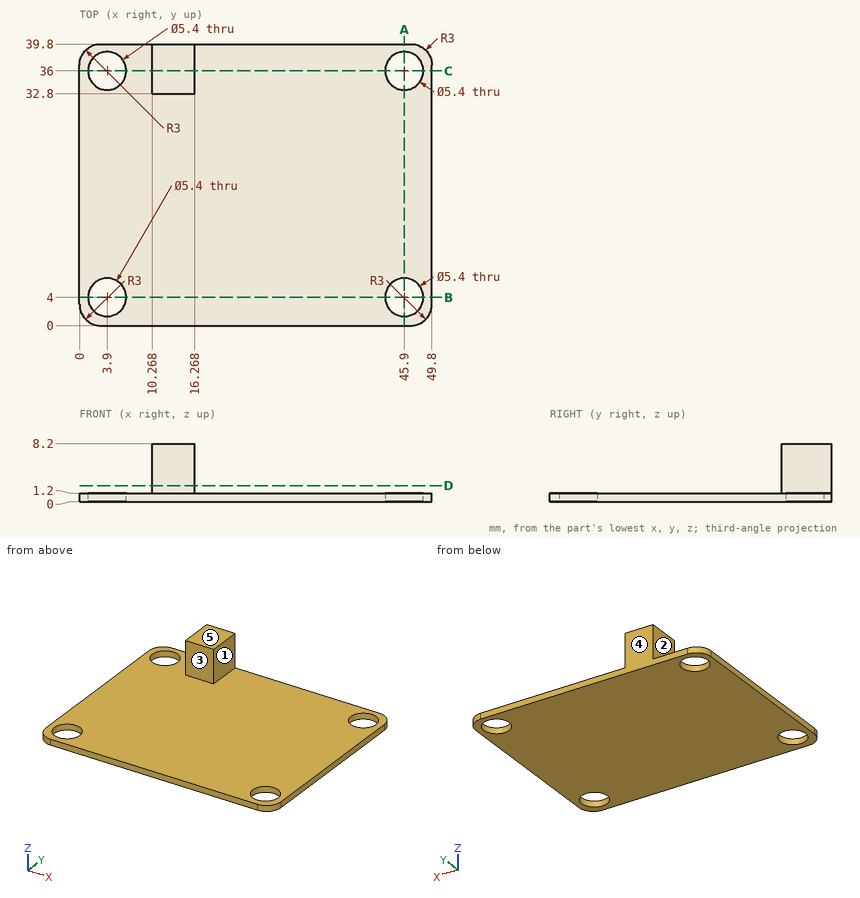
Source: three-view drawing plus pictorial views. Frame: mm from the lowest corner of the part. A direction names the side the tool comes from. Give positions to 0.01 mm unless a question says otherwise; leave off trailing zeros. Order: outer loops, then holes, each group sorted by start corner. A loop starts at its lowest first (then second) coordinate and runs counter-clockwise, first axis right, second up. Notation, with made-up numbers: (31, 89) -> (47, 89) arc R19 cw to (47, 93) -> close; hole circle Ø10 at (83.25, -5.75). An arc over 180 degrees is marked (long way). Use a Markdown table: item, result.
Q1. First-contact query: P1, Ø20, axis at x = 27, y = 27.5, coming from the +Z side; P2, Ø4.5, axis at x = 45.9, y = 36, coming from the -Z side; P3, Ø3, axis at x = 11.5, z = 6.5, coming from the -Y side; P4, Ø3.5, axis at y = 37, z = 3, coming from the -X side. Flat tips, straight axial feed; report the tip coordinate or a pass-through.
A:
| item | result |
|---|---|
| P1 | z = 1.2 |
| P2 | through |
| P3 | y = 32.8 |
| P4 | x = 10.27 |
Q2. Material intervals for line 1 (Y direction, x = 45.9, z = 0.7); line 2 (Y direction, x = 47, z = 1); line 3 (Z direction, x = 22.5, y = 7.5), sorted ascending. Write a range as [from, to].
A:
| item | result |
|---|---|
| line 1 | [0, 1.3], [6.7, 33.3], [38.7, 39.8] |
| line 2 | [0.01, 1.53], [6.47, 33.53], [38.47, 39.79] |
| line 3 | [0, 1.2] |
Q3. Section D-D (z = 2.25). Return the cut outline in (x, y), and give its area (3 significant figures).
A:
| item | result |
|---|---|
| outline | (10.27, 32.8) -> (16.27, 32.8) -> (16.27, 39.8) -> (10.27, 39.8) -> close |
| area | 42.0 mm^2 |
Q4. Section A-A (x = 45.9). Return the cut outline in (y, z), and give its area (3 significant figures).
A:
| item | result |
|---|---|
| outline | (0, 0) -> (1.3, 0) -> (1.3, 1.2) -> (0, 1.2) -> close; (6.7, 0) -> (33.3, 0) -> (33.3, 1.2) -> (6.7, 1.2) -> close; (38.7, 0) -> (39.8, 0) -> (39.8, 1.2) -> (38.7, 1.2) -> close |
| area | 34.8 mm^2 |
Q5. Section C-C (y = 36). Return the cut outline in (x, z), and give its area (3 significant figures).
A:
| item | result |
|---|---|
| outline | (0, 0) -> (1.2, 0) -> (1.2, 1.2) -> (0, 1.2) -> close; (6.6, 0) -> (43.2, 0) -> (43.2, 1.2) -> (16.27, 1.2) -> (16.27, 8.2) -> (10.27, 8.2) -> (10.27, 1.2) -> (6.6, 1.2) -> close; (48.6, 0) -> (49.8, 0) -> (49.8, 1.2) -> (48.6, 1.2) -> close |
| area | 88.8 mm^2 |
Q6. Section B-B (y = 4). Return the cut outline in (x, z), and give its area (3 significant figures).
A:
| item | result |
|---|---|
| outline | (0, 0) -> (1.2, 0) -> (1.2, 1.2) -> (0, 1.2) -> close; (6.6, 0) -> (43.2, 0) -> (43.2, 1.2) -> (6.6, 1.2) -> close; (48.6, 0) -> (49.8, 0) -> (49.8, 1.2) -> (48.6, 1.2) -> close |
| area | 46.8 mm^2 |
Q7. Access query for the marked faces 1, 2, 3, 4 and 5. Directions: +Z, -Z, +X, -X, +Y, -Y. A direction counts if a zero-diameter tool reaches every point of the face in a straight line with its end or side. Return the directions, or none.
A:
| item | result |
|---|---|
| face 1 | +Z, +X, +Y, -Y |
| face 2 | +Z, -X, +Y, -Y |
| face 3 | +Z, +X, -X, -Y |
| face 4 | +Z, -Z, +X, -X, +Y |
| face 5 | +Z, +X, -X, +Y, -Y |
